from build123d import *

# Parameters (mm, degrees)
SKETCH1_R                   = 15
BOSS_EXTRUDE1_DEPTH         = 10
SKETCH2_R                   = 0.484915
CUT_EXTRUDE1_DEPTH          = 10
CIRPATTERN1_COUNT           = 4
SKETCH7_R                   = 1.44135
CUT_EXTRUDE2_DEPTH          = 24.34691072
CIRPATTERN2_COUNT           = 4
CIRPATTERN2_COPY_1_SKETCH_R = 1.44135
CIRPATTERN2_COPY_1_DEPTH    = 24.34691072
CIRPATTERN2_COPY_2_SKETCH_R = 1.44135
CIRPATTERN2_COPY_2_DEPTH    = 24.34691072
CIRPATTERN2_COPY_3_SKETCH_R = 1.44135
CIRPATTERN2_COPY_3_DEPTH    = 24.34691072


with BuildPart() as part:
    # Sketch1 → Boss-Extrude1 (new body)
    with BuildSketch(Plane.XY):
        Circle(SKETCH1_R)
    extrude(amount=BOSS_EXTRUDE1_DEPTH)

    # Sketch2 → Cut-Extrude1 (cut)
    with BuildSketch(Plane.XY.offset(10)):
        with Locations((2.828427125, 2.828427125)):
            Circle(SKETCH2_R)
    cut_extrude1 = extrude(amount=-CUT_EXTRUDE1_DEPTH, mode=Mode.SUBTRACT)

    # CirPattern1: Cut-Extrude1 ×4 about axis
    cirpattern1_axis = Axis((0, 0, 0), (0, 0, 1))
    for i in range(1, CIRPATTERN1_COUNT):
        add(cut_extrude1.rotate(cirpattern1_axis, i * 360 / CIRPATTERN1_COUNT), mode=Mode.SUBTRACT)

    # Sketch7 → Cut-Extrude2 (cut, symmetric)
    with BuildSketch(Plane(origin=(-0.025287604, 0.006355569, 0.298027772), x_dir=(0.2437507452891652, 0.9698379112877453, 0), z_dir=(0.08452694350312104, -0.02124427725097248, -0.9961946980917455))):
        with Locations(Location((2.053684635, -7.185898346, 0), (0, 0, 90))):
            Circle(SKETCH7_R)
    cut_extrude2 = extrude(amount=CUT_EXTRUDE2_DEPTH, both=True, mode=Mode.SUBTRACT)

    # Mirror1: Cut-Extrude2 across plane
    add(cut_extrude2.mirror(Plane(origin=(0, 0, 0), x_dir=(0, 0, 1), z_dir=(-0.7071067811865512, -0.7071067811865438, 0))), mode=Mode.SUBTRACT)

    # CirPattern2: Cut-Extrude2 ×4 about axis
    cirpattern2_axis = Axis((0, 0, 10), (0, 0, -1))
    for i in range(1, CIRPATTERN2_COUNT):
        add(cut_extrude2.rotate(cirpattern2_axis, i * 360 / CIRPATTERN2_COUNT), mode=Mode.SUBTRACT)

    # CirPattern2 copy 1 sketch → CirPattern2 copy 1 (cut, symmetric)
    with BuildSketch(Plane(origin=(0.025287604, 0.006355569, 0.298027772), x_dir=(-0.24375074528915505, 0.9698379112877479, 0), z_dir=(-0.08452694350312126, -0.021244277250971604, -0.9961946980917455))):
        with Locations((2.053684635, 7.185898346)):
            Circle(CIRPATTERN2_COPY_1_SKETCH_R)
    extrude(amount=CIRPATTERN2_COPY_1_DEPTH, both=True, mode=Mode.SUBTRACT)

    # CirPattern2 copy 2 sketch → CirPattern2 copy 2 (cut, symmetric)
    with BuildSketch(Plane(origin=(0.006355569, -0.025287604, 0.298027772), x_dir=(0.9698379112877479, 0.2437507452891551, 0), z_dir=(-0.02124427725097161, 0.08452694350312126, -0.9961946980917455))):
        with Locations((2.053684635, 7.185898346)):
            Circle(CIRPATTERN2_COPY_2_SKETCH_R)
    extrude(amount=CIRPATTERN2_COPY_2_DEPTH, both=True, mode=Mode.SUBTRACT)

    # CirPattern2 copy 3 sketch → CirPattern2 copy 3 (cut, symmetric)
    with BuildSketch(Plane(origin=(-0.025287604, -0.006355569, 0.298027772), x_dir=(0.24375074528915516, -0.9698379112877479, 0), z_dir=(0.08452694350312126, 0.021244277250971614, -0.9961946980917455))):
        with Locations((2.053684635, 7.185898346)):
            Circle(CIRPATTERN2_COPY_3_SKETCH_R)
    extrude(amount=CIRPATTERN2_COPY_3_DEPTH, both=True, mode=Mode.SUBTRACT)


solid = part.part
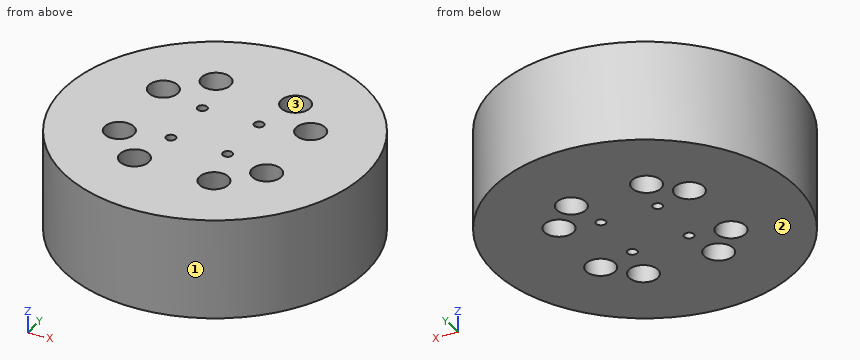
The model under review builds one solid part; all positions refer to its coordinate system, in mm. Face numbers are marked on the shaded views. Coordinates: 2 decimals unless noted, no trailing zeros. Write each loop counter-clockwise with the first axis right and the second up, starting at its lowest first coordinate (ties: lowest second). Pieces come first, ordered by that corner, then holes. Notation, with made-up numbers: (37, 7) -> (59, 7) arc R26 ccw to (59, 29) -> close; hole circle Ø9 at (-17.75, 58). An arc over 180 degrees is marked (long way). Answer in a Markdown table with one row per item.
1. Wall thickness on probe 1 along Y at (x, z) = (-3, 9.75); probe 2 along Y at (x, z) = (7, 0.5); probe 3 along X at (y, z) = (5, 4): over which ranges is each line inside the solid? List them lowest first. Write a range as [from, to].
Answers below:
| item | result |
|---|---|
| probe 1 | y = [-14.7, -8.4], [-6.24, -3.28], [-2.37, 2.37], [3.28, 6.24], [8.4, 14.7] |
| probe 2 | y = [-13.27, -5.13], [-2.4, 2.4], [5.13, 13.27] |
| probe 3 | x = [-14.14, -7.69], [-5.98, 5.98], [7.69, 14.14] |
2. Draft analysis for pull direction Y (two halves, no side actions). For the marked faces 1, 2 and 3, state which applies: +Y half, -Y half, draft (parallel to the pull), parting line (faces both ways), or undercut.
Answers below:
| item | result |
|---|---|
| face 1 | parting line |
| face 2 | draft |
| face 3 | undercut |
3. We need section B-B, the plane y = 10. State the section outline as (x, z) points, and give its area (3 significant figures).
Answers below:
| item | result |
|---|---|
| outline | (-11.18, 0) -> (11.18, 0) -> (11.18, 10) -> (-11.18, 10) -> close |
| area | 224 mm^2 |
4. We need section A-A, the plane z = 6.5. Give the number of separate pieces and of enclosed holes in the cut face, and give its area (3 significant figures).
Answers below:
| item | result |
|---|---|
| separate pieces | 1 |
| enclosed holes | 12 |
| area | 651 mm^2 |
5. Clearance check with flat-ended pins moving along their axes: pin 1 Ø1.5 at (y, z) = (11.5, 1.5) entering from +X; pin 2 Ø3 at (x, z) = (2.5, 5.5) entering from +Y; pin 3 Ø1 at (y, z) = (-6.5, 1.5) entering from +X. State where each tip first meets the part, or that it passes through.
Answers below:
| item | result |
|---|---|
| pin 1 | stops at x = 10.46 |
| pin 2 | stops at y = 14.97 |
| pin 3 | stops at x = 13.75 |
